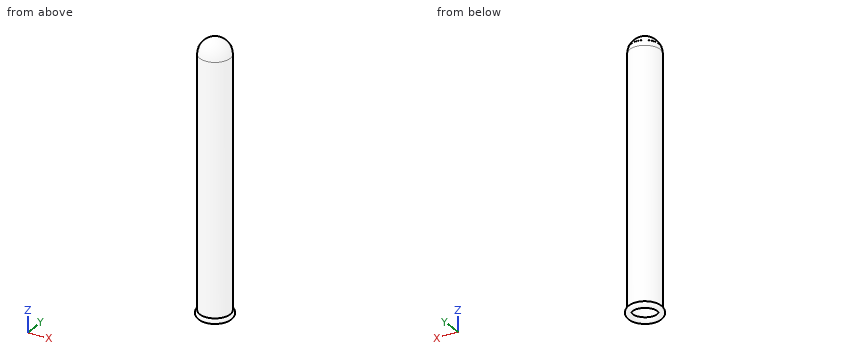
```python
from build123d import *

# Parameters (mm, degrees)
SKETCH40_R          = 8
BOSS_EXTRUDE4_DEPTH = 140
SKETCH41_R          = 7.5
CUT_EXTRUDE3_DEPTH  = 135
FILLET5_R           = 8


# Read off the part's stored shape, not the designer's step: Sweep3
with BuildPart() as part:
    # Sketch40 → Boss-Extrude4 (new body)
    with BuildSketch(Plane.XY):
        Circle(SKETCH40_R)
    extrude(amount=BOSS_EXTRUDE4_DEPTH)

    # Sketch41 → Cut-Extrude3 (cut)
    with BuildSketch(Plane(origin=(0, 0, 0), x_dir=(-1, 0, 0), z_dir=(0, 0, -1))):
        Circle(SKETCH41_R)
    extrude(amount=-CUT_EXTRUDE3_DEPTH, mode=Mode.SUBTRACT)

    # Sweep3 outline → Sweep3 (revolve)
    with BuildSketch(Plane.XZ):
        with BuildLine():
            Line((8, 1.414213562), (8, 0))
            Line((8, 0), (7.5, 0))
            Line((7.5, 0), (7.5, 1.5))
            ThreePointArc((7.5, 1.5), (7.24634703, -1.478397839), (8, 1.414213562))
        make_face()
    revolve(axis=Axis((0, 0, 0), (0, 0, 1)))

    # Fillet5
    fillet5_edges = [part.edges().sort_by_distance(p)[0] for p in [
        (-8, 0, 140),
    ]]
    fillet(fillet5_edges, radius=FILLET5_R)


solid = part.part
```
The listing builds one solid part. Answer for the finished solid, in the listing's coordinates (mm). Give positions to 0.01 mm unless a question says otherwise; leave off trailing zeros. Order: outer loops, then holes, each group sorted by start corner. A loop starts at its lowest first (then second) coordinate and runs counter-clockwise, first axis right, second up. Notation, with made-up numbers: (86.5, 79.25) -> (128.5, 79.25) arc R27 cw to (128.5, 98.25) -> close; hole circle Ø5 at (-18.75, 76.5). An arc over 180 degrees is marked (long way). One line per item, written item: value.
1) Find section B-B, the plane z = 110.5. Determine the outline of the cut face in (x, y).
Reported:
outline: circle Ø16 at (0, 0); hole circle Ø15 at (0, 0)
2) Flat-ended cylindrical pins translate along their axes: P1, Ø9, axis at x = 0, y = 0, coming from the -Z side; P2, Ø3, axis at x = -4, z = 45.5, coming from the +Y side; P3, Ø1, axis at y = -5, z = 108.5, coming from the -X side. Find the tip coordinate at first contact, or state that the pin passes through.
Reported:
P1: stops at z = 135
P2: stops at y = 7.6
P3: stops at x = -6.61
3) Find the intervals of material crossed by line 1 (X direction, y = 0.25, z = 61); line 2 (Z direction, x = 6.25, y = -0.75), in increasing order.
Reported:
line 1: x = -8 to -7.5, 7.5 to 8
line 2: z = -0.89 to 0.89, 135 to 136.94
